CAD build for the part. Positions are in the model's coordinates, mm. A direction names the side the tool comes from. Coordinates: 2 decimals unless noted, no trailing zeros. Loops run counter-clockwise (first coordinate to the right, second up) from the corner with the lowest first, then second, coordinate; pieces in that order, holes last.
1) Which spindle directions (+Z, -Z, +X, -X, +Y, -Y) get a long thin tool onto all of the face, cutting with end or side? Do faces 1 (the cylindrical face through (6.81, 1.438, 0.748)), 2 (the flat face through (0, 2, -2)). Say none if no direction does.
2) Two-plate mould, pull along Y, no slides. Class faces 3 (the cylindrical face through (38.525, -0.867, -3.905)), 4 (the flat face through (76, 2, -2)), 5 (the conical face through (62, 0, 0)), 6 (the cylindrical face through (69.19, 1.438, -0.748)): +Y half, -Y half, draft (parallel to the pull), parting line (faces both ways), or undercut.
3) Saw through at A-A, the plane x = 71.5. Write the cut outline in (y, z), and give its area (3 significant figures).
4) Saw through at B-B, the plane x = 52. Write the cut outline in (y, z).
5) Wall check: line 1 along Z through (x, y) = (71, 0); line 2 along X through (y, z) = (0.25, -3.5); line 3 along Y through (x, z) = (63, -0.5). Give the ranges that are in metal, low to high.
6) Pin check, flat tips, straight feed: pin 1 Ø1 at (y, z) = (3, -2.5) entering from -X; pin 2 Ø1.5 at (x, y) = (59.5, 2.5) entering from -Z; pin 3 Ø1 at (x, y) = (13, -1.5) entering from +Z. Stop position of each tip, or through.
Autodesk Inventor part; units mm, degrees
ref_plane "YZ Plane" through (0, 0, 0) normal (1, 0, 0) x (0, 1, 0)
ref_plane "XZ Plane" through (0, 0, 0) normal (0, 1, 0) x (-1, 0, 0)
ref_plane "XY Plane" through (0, 0, 0) normal (0, 0, 1) x (1, 0, 0)
sketch "Sketch_1" plane through (0, 0, 0) normal (0, 0, 1) x (1, 0, 0)
  line L0 (76, 0) -> (0, 0)
  line L1 (0, 0) -> (0, 3.5)
  line L2 (0, 3.5) -> (0.5, 4)
  line L3 (0.5, 4) -> (75.5, 4)
  line L4 (75.5, 4) -> (76, 3.5)
  line L5 (76, 3.5) -> (76, 0)
  line L6 (76, 0) -> (0, 0)
revolve "Revolution1" add sketch "Sketch_1" angle 360 about axis through (76, 0, 0) along (1, 0, 0)
sketch "Sketch2" plane through (0, 0, 0) normal (-1, 0, 0) x (0, 0, 1)
  point P0 (0, 0)
hole "Hole1" at (0, 0, 0) direction (1, 0, 0) diameter 3.242 depth 13.0641 tip angle 120 countersink diameter 4 countersink angle 90
sketch "Sketch3" plane through (76, 0, 0) normal (1, 0, 0) x (0, 0, -1)
  point P0 (0, 0)
hole "Hole2" at (76, 0, 0) direction (-1, 0, 0) diameter 3.242 depth 13.0641 tip angle 120 countersink diameter 4 countersink angle 90
properties part number "SFHRW8-76-M4-N4" material "鋼、炭素鋼"
Data:
1. face 1: -X
1. face 2: +Z, -Z, -X, +Y, -Y
2. face 3: parting line
2. face 4: draft
2. face 5: undercut
2. face 6: undercut
3. outline: circle Ø8 at (0, 0); hole circle Ø3.24 at (0, 0)
3. area: 42.0 mm2
4. outline: circle Ø8 at (0, 0)
5. line 1: z = -4 to -1.62, 1.62 to 4
5. line 2: x = 0.01 to 75.99
5. line 3: y = -3.97 to -1.54, 1.54 to 3.97
6. pin 1: stops at x = 0
6. pin 2: stops at z = -3.6
6. pin 3: stops at z = 3.87
